```python
from build123d import *

# Parameters (mm, degrees)
SKETCH1_R           = 38.1
BOSS_EXTRUDE1_DEPTH = 6.35
CUT_EXTRUDE1_DEPTH  = 7.35
FILLET1_R           = 0.762
CUT_EXTRUDE3_DEPTH  = 7.35


with BuildPart() as part:
    # Sketch1 → Boss-Extrude1 (new body)
    with BuildSketch(Plane.XY):
        Circle(SKETCH1_R)
    extrude(amount=BOSS_EXTRUDE1_DEPTH)

    # Sketch2 → Cut-Extrude1 (cut, through all)
    with BuildSketch(Plane.XY.offset(6.35)):
        with BuildLine():
            Line((-4.8895, 33.2105), (-4.8895, 37.784954542))
            ThreePointArc((-4.8895, 37.784954542), (0, 38.1), (4.8895, 37.784954542))
            Line((4.8895, 37.784954542), (4.8895, 33.2105))
            ThreePointArc((4.8895, 33.2105), (0, 28.321), (-4.8895, 33.2105))
        make_face()
        with BuildLine():
            Line((31.205886672, -12.370818788), (35.167480514, -14.658046059))
            ThreePointArc((35.167480514, -14.658046059), (32.995567884, -19.05), (30.277980514, -23.126908483))
            Line((30.277980514, -23.126908483), (26.316386672, -20.839681212))
            ThreePointArc((26.316386672, -20.839681212), (24.526705461, -14.1605), (31.205886672, -12.370818788))
        make_face()
        with BuildLine():
            Line((-26.316386672, -20.839681212), (-30.277980514, -23.126908483))
            ThreePointArc((-30.277980514, -23.126908483), (-32.995567884, -19.05), (-35.167480514, -14.658046059))
            Line((-35.167480514, -14.658046059), (-31.205886672, -12.370818788))
            ThreePointArc((-31.205886672, -12.370818788), (-24.526705461, -14.1605), (-26.316386672, -20.839681212))
        make_face()
    extrude(amount=-CUT_EXTRUDE1_DEPTH, mode=Mode.SUBTRACT)

    # Fillet1
    fillet1_edges = [part.edges().sort_by_distance(p)[0] for p in [
        (-4.8895, 37.784954542, 3.175),
        (4.8895, 37.784954542, 3.175),
        (35.167480514, -14.658046059, 3.175),
        (30.277980514, -23.126908483, 3.175),
        (-30.277980514, -23.126908483, 3.175),
        (-35.167480514, -14.658046059, 3.175),
    ]]
    fillet(fillet1_edges, radius=FILLET1_R)

    # Sketch4 → Cut-Extrude3 (cut, through all)
    with BuildSketch(Plane.XY.offset(6.35)):
        with BuildLine():
            Line((-1.9558, -1.62063147), (-1.9558, 1.62063147))
            ThreePointArc((-1.9558, 1.62063147), (2.54, 0), (-1.9558, -1.62063147))
        make_face()
    extrude(amount=-CUT_EXTRUDE3_DEPTH, mode=Mode.SUBTRACT)


solid = part.part
```
Check sheet for the modelled part. Datum: model origin and axes. Units: mm. A direction names the side the tool comes from. Give positions to 0.01 mm unless a question says otherwise; leave off trailing zeros. Order: outer loops, then holes, each group sorted by start corner. A loop starts at its lowest first (then second) coordinate and runs counter-clockwise, first axis right, second up. Notation, with made-up numbers: M 20,64 L 72,64 A13 cw 72,80 Z; hole C 89,22 d4. An arc over 180 degrees is marked long. Answer in a Markdown table with one row per item. Add a question column.
Q1. Gauge pin test, flat ends, axial feed: pin 1 Ø3 at (x, z) = (-11, 5) entering from +Y; pin 2 Ø3 at (y, z) = (5, 4) entering from -X; pin 3 Ø1.8 at (y, z) = (34, 3.5) entering from +X. Record the tip position at first contact, or that the pin passes through.
Q2. Sectioned sample at C-C, the plane x = 0. Record the boundary of the cut face in (y, z), and give its area (3 significant figures).
Q3. Sectioned sample at A-A, the plane z = 2. Record the boundary of the cut face in (x, y).
Q4. Access from +Z, -Z, +X, -X, +Y, -Y to the whole of each face (thin tool, end or side, straight path). Record for faces 5 (the flat face through (-27.89, -21.75, 3.22)), 6 (the flat face through (-32.83, -13.31, 3.22)), 7 (the flat face through (4.89, 35, 3)), 8 (the flat face through (27.94, -21.777, 3.219)).
Q5. Sectioned sample at D-D, the plane x = -10. Record the boundary of the cut face in (y, z), and give its area (3 significant figures).
Q6. Sectioned sample at B-B, the plane y = 0. Record the boundary of the cut face in (x, z), and give its area (3 significant figures).
Q7. Release check for a two-part mould opening along Y. For faces 1 (the flat face through (-1.956, 0, 3)), 2 (the flat face through (32.78, -13.28, 3.22)), 3 (the flat face through (8, 0, 0)), 4 (the cylindrical face through (0.108, 28.322, 3.219)) record: released by +Y, released by -Y, zero draft, split by the parting line, or undercut.
Q8. Thickness scan on L1, parallel to Y at x = 0, z = 3; L2, parallel to X at y = -12.5, z = 2.25; L3, parallel to Y at x = -29.5, z = 6.25. Record the ranges inside material, lowest first.
Verdict:
| question | item | result |
|---|---|---|
| 1 | pin 1 | y = 36.9 |
| 1 | pin 2 | x = -37.94 |
| 1 | pin 3 | x = 18.87 |
| 2 | outline | M -38.1,0 L -2.54,0 L -2.54,6.35 L -38.1,6.35 Z; M 2.54,0 L 28.32,0 L 28.32,6.35 L 2.54,6.35 Z |
| 2 | area | 390 mm² |
| 3 | outline | M -35.5,-13.84 A0.76 ccw -34.41,-14.22 L -31.21,-12.37 A4.89 cw -26.32,-20.84 L -29.52,-22.69 A0.76 ccw -29.73,-23.82 A38.1 ccw 29.73,-23.82 A0.76 ccw 29.52,-22.69 L 26.32,-20.84 A4.89 cw 31.21,-12.37 L 34.41,-14.22 A0.76 ccw 35.5,-13.84 A38.1 ccw 5.77,37.66 A0.76 ccw 4.89,36.91 L 4.89,33.21 A4.89 cw -4.89,33.21 L -4.89,36.91 A0.76 ccw -5.77,37.66 A38.1 ccw Z; hole M -1.96,-1.62 A2.54 ccw long -1.96,1.62 Z |
| 4 | face 5 | +Z, -Z, -X |
| 4 | face 6 | +Z, -Z, -Y |
| 4 | face 7 | +Z, -Z, +Y |
| 4 | face 8 | +Z, -Z, +X |
| 5 | outline | M -36.76,0 L 36.76,0 L 36.76,6.35 L -36.76,6.35 Z |
| 5 | area | 467 mm² |
| 6 | outline | M -38.1,0 L -1.96,0 L -1.96,6.35 L -38.1,6.35 Z; M 2.54,0 L 38.1,0 L 38.1,6.35 L 2.54,6.35 Z |
| 6 | area | 455 mm² |
| 7 | face 1 | undercut |
| 7 | face 2 | released by -Y |
| 7 | face 3 | zero draft |
| 7 | face 4 | released by +Y |
| 8 | L1 | -38.1 to -2.54, 2.54 to 28.32 |
| 8 | L2 | -35.99 to -31.43, -26.11 to 26.11, 31.43 to 35.99 |
| 8 | L3 | -24.11 to -22.68, -11.77 to 24.11 |
